Here's how the part is built. I have some questions about the finished solid (model axes, mm). A direction names the side the tool comes from. Give positions to 0.01 mm unless a question says otherwise; leave off trailing zeros. Write each loop counter-clockwise with the first axis right and the second up, starting at its lowest first coordinate (ties: lowest second). Pieces come first, ordered by that corner, then holes. Notation, with made-up numbers: (-15.75, 60) -> (2.25, 60) arc R13 ccw to (2.25, 71) -> close; hole circle Ø1 at (75.5, 68). An arc over 180 degrees is marked (long way). Return JSON: item names as keys, results as strings.
from build123d import *

# Parameters (mm, degrees)
CROQUIS2_R            = 7.742665811
CORTAR_EXTRUIR1_DEPTH = 14.272066445
CHAFL_N1_SIZE         = 0.2


with BuildPart() as part:
    # Croquis1 → Revolución1 (revolve)
    with BuildSketch(Plane.XY, mode=Mode.PRIVATE) as revoluci_n1_sk:
        Polygon((0.2, 0), (0.5, 0), (7.742665811, 7.5), (2.75, 7.5), (2.75, 13.5), (1.6, 13.5), (1.6, 2.424871131), align=None)
    revolve(revoluci_n1_sk.sketch.rotate(Axis((0, 0, 0), (0, 1, 0)), 270), axis=Axis((0, 0, 0), (0, 1, 0)))

    # Croquis2 → Cortar-Extruir1 (cut, through all)
    with BuildSketch(Plane(origin=(0, 7.5, 0), x_dir=(1, 0, 0), z_dir=(0, 1, 0))):
        Circle(CROQUIS2_R)
        Polygon((2.309401077, 4), (-2.309401077, 4), (-4.618802154, 0), (-2.309401077, -4), (2.309401077, -4), (4.618802154, 0), align=None, mode=Mode.SUBTRACT)
    extrude(amount=-CORTAR_EXTRUIR1_DEPTH, mode=Mode.SUBTRACT)

    # Chaflán1
    chafl_n1_edges = [part.edges().sort_by_distance(p)[0] for p in [
        (0, 13.5, -1.6),
    ]]
    chamfer(chafl_n1_edges, length=CHAFL_N1_SIZE)


solid = part.part
1. Suppose I cut it at B-B, the plane y = 11.5. List the corners of the cut face in (x, z) for me.
Taken from the geometry:
{"outline": "circle Ø5.5 at (0, 0); hole circle Ø3.2 at (0, 0)"}
2. If we mould it in two halves opening along X, with no side actions, what happens to faces 3 (the face through (3.48, 5.59, -1.97)), 4 (the face through (-0.72, 0.93, -0.16)), 5 (the face through (0, 6, 4))? For each: released by +X, released by -X, zero draft, split by the parting line, or undercut.
Taken from the geometry:
{"face 3": "released by +X", "face 4": "undercut", "face 5": "zero draft"}
3. Suppose I cut it at C-C, the plane y = 2. List the corners of the cut face in (x, z) for me, and give its area (3 significant figures).
Taken from the geometry:
{"outline": "circle Ø4.86 at (0, 0); hole circle Ø2.71 at (0, 0)", "area": "12.8 mm²"}
4. If I drill on line 1 (X direction, y = 10.25, z = 0); line 2 (Z direction, x = 1, y = 12.5); line 3 (Z direction, x = 0.5, y = 2.5), over which ranges is the centre line in solid material (lowest first)? Write a range as [from, to].
Taken from the geometry:
{"line 1": "x = [-2.75, -1.6], [1.6, 2.75]", "line 2": "z = [-2.56, -1.25], [1.25, 2.56]", "line 3": "z = [-2.87, -1.52], [1.52, 2.87]"}
5. Which directions (+Z, -Z, +X, -X, +Y, -Y) give clear straight access to the entire face, cutting with the end or side of a thin tool? Please do faces 1 (the face through (-2.685, 10.542, -0.596)), 2 (the face through (-3.448, 5.589, -2.028)).
Taken from the geometry:
{"face 1": "+Y", "face 2": "-Z, -X, +Y, -Y"}
6. Suppose I cut it at A-A, the plane x = 0. List the corners of the cut face in (y, z) for me.
Taken from the geometry:
{"outline": "(0, -0.5) -> (3.62, -4) -> (7.5, -4) -> (7.5, -2.75) -> (13.5, -2.75) -> (13.5, -1.8) -> (13.3, -1.6) -> (2.42, -1.6) -> (0, -0.2) -> close; (0, 0.2) -> (2.42, 1.6) -> (13.3, 1.6) -> (13.5, 1.8) -> (13.5, 2.75) -> (7.5, 2.75) -> (7.5, 4) -> (3.62, 4) -> (0, 0.5) -> close"}
7. For pin 1 Ø1 at (x, y) = (-3, 9) entering from -Z; pin 2 Ø1 at (y, z) = (6, -1.5) entering from -X; pin 3 Ø1.5 at (x, y) = (-3.5, 5) entering from -Z, each with a flat end and sliding along its axis, tell me the tip position at first contact or that it passes through.
Taken from the geometry:
{"pin 1": "stops at z = -1.15", "pin 2": "stops at x = -4.04", "pin 3": "stops at z = -3.24"}
